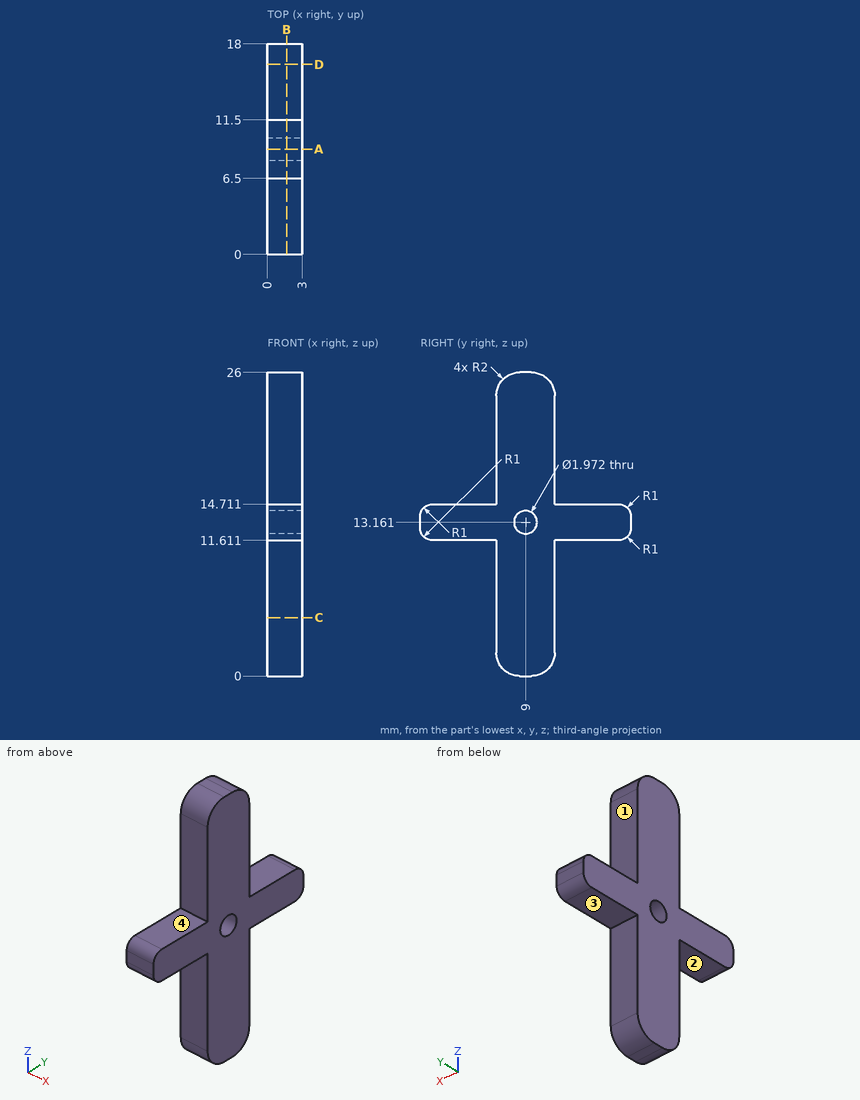
Here's the drawing with two shaded views (mm, measured from the low corner). I have some questions. A direction names the side the tool comes from. Round coordinates to 2 decimals unless told otherwise and drop trailing zeros. Write each loop counter-clockwise with the first axis right and the second up, starting at its lowest first coordinate (ties: lowest second). Pieces come first, ordered by that corner, then holes. Notation, with made-up numbers: M 14.25,53.5 L 32.25,53.5 A18 ccw 32.25,85.5 Z; hole C -10.5,33.25 d5. An arc over 180 degrees is marked long. Answer in a Markdown table with one row per item. Add a question column.
Q1. If I drill on line 1 (Z direction, x = 2.2, y = 9) (1 decimal); line 2 (Y direction, x = 2.45, z = 13.25); line 3 (Y direction, x = 0.3, z = 19), over which ranges is the centre line in solid material (lowest first)? Write a range as from..to.
Q2. Imagine slicing it at C-C (z = 5). Please give me the cut outline in (x, y), then the cut area to 3 significant figures.
Q3. On a 3-axis mill with a long thin cutter (end or side, diameter ignored), from which of +Z, -Z, +X, -X, +Y, -Y can I reach the whole of each face in a straight line? I mean the marked faces 1, 2, 3 and 4. Say none if no direction works.
Q4. Imagine slicing it at B-B (x = 1.65). Please give me the cut outline in (y, z) (1 decimal).
Q5. Will these pins go through, and if not, where does the flat tip stop? pin 1 Ø5 at (y, z) = (12.5, 8) entering from +X; pin 2 Ø0.9 at (x, z) = (1, 17.5) entering from -Y; pin 3 Ø0.9 at (x, z) = (2, 17.5) entering from +Y; pin 4 Ø1.5 at (x, y) = (1.5, 2.5) entering from -Z.
Q6. Imagine slicing it at D-D (y = 16.25). Please give me the cut outline in (x, z).
Q7. Imagine slicing it at A-A (y = 9). Please give me the cut outline in (x, z) (1 decimal).
Values:
| question | item | result |
|---|---|---|
| 1 | line 1 | 0..12.2, 14.1..26 |
| 1 | line 2 | 0..8.02, 9.98..18 |
| 1 | line 3 | 6.5..11.5 |
| 2 | outline | M 0,6.5 L 3,6.5 L 3,11.5 L 0,11.5 Z |
| 2 | area | 15.0 mm^2 |
| 3 | face 1 | +Z, +X, -X, +Y |
| 3 | face 2 | -Z, +X, -X, -Y |
| 3 | face 3 | -Z, +X, -X, +Y |
| 3 | face 4 | +Z, +X, -X, -Y |
| 4 | outline | M 0,12.6 A1 ccw 1,11.6 L 6.5,11.6 L 6.5,2 A2 ccw 8.5,0 L 9.5,0 A2 ccw 11.5,2 L 11.5,11.6 L 17,11.6 A1 ccw 18,12.6 L 18,13.7 A1 ccw 17,14.7 L 11.5,14.7 L 11.5,24 A2 ccw 9.5,26 L 8.5,26 A2 ccw 6.5,24 L 6.5,14.7 L 1,14.7 A1 ccw 0,13.7 Z; hole C 9,13.2 d2 |
| 5 | pin 1 | x = 3 |
| 5 | pin 2 | y = 6.5 |
| 5 | pin 3 | y = 11.5 |
| 5 | pin 4 | z = 11.61 |
| 6 | outline | M 0,11.61 L 3,11.61 L 3,14.71 L 0,14.71 Z |
| 7 | outline | M 0,0 L 3,0 L 3,12.2 L 0,12.2 Z; M 0,14.1 L 3,14.1 L 3,26 L 0,26 Z |
